```python
from build123d import *

# Parameters (mm, degrees)
SKETCH1_R           = 2.075
SKETCH1_R_2         = 6.003208263
BOSS_EXTRUDE2_DEPTH = 8
FILLET1_R           = 2
CUT_EXTRUDE1_DEPTH  = 10
FILLET2_R           = 2
CUT_EXTRUDE2_DEPTH  = 10
FILLET3_R           = 2


with BuildPart() as part:
    # Sketch1 → Boss-Extrude2 (new body)
    with BuildSketch(Plane(origin=(0, 0, 0), x_dir=(1, 0, 0), z_dir=(0, 1, 0))):
        with BuildLine():
            Line((0, 44.83), (0, 36.83))
            ThreePointArc((0, 36.83), (36.83, 0), (0, -36.83))
            Line((0, -36.83), (0, -46.83))
            Line((0, -46.83), (0, -58.83))
            ThreePointArc((0, -58.83), (14.116701064, -87.229775601), (8, -56.110417137))
            Line((8, -56.110417137), (8, -44.110417137))
            ThreePointArc((8, -44.110417137), (44.649741882, 4.016148637), (0, 44.83))
        make_face()
        with Locations(Location((0.96696537, -64.081170969, 0), (0, 0, 270))):
            Circle(SKETCH1_R, mode=Mode.SUBTRACT)
        with Locations(Location((16.96696537, -64.081170969, 0), (0, 0, 270))):
            Circle(SKETCH1_R, mode=Mode.SUBTRACT)
        with Locations(Location((16.96696537, -80.081170969, 0), (0, 0, 270))):
            Circle(SKETCH1_R, mode=Mode.SUBTRACT)
        with Locations(Location((0.96696537, -80.081170969, 0), (0, 0, 270))):
            Circle(SKETCH1_R, mode=Mode.SUBTRACT)
        with Locations(Location((8.96696537, -72.081170969, 0), (0, 0, 270))):
            Circle(SKETCH1_R_2, mode=Mode.SUBTRACT)
    extrude(amount=BOSS_EXTRUDE2_DEPTH)

    # Fillet1
    fillet1_edges = [part.edges().sort_by_distance(p)[0] for p in [
        (0, 4, 58.83),
        (0, 4, 36.83),
        (0, 4, -36.83),
        (0, 4, -44.83),
        (8, 4, 44.110417137),
        (8, 4, 56.110417137),
    ]]
    fillet(fillet1_edges, radius=FILLET1_R)

    # Sketch2 → Cut-Extrude1 (cut)
    with BuildSketch(Plane(origin=(0, 8, 0), x_dir=(1, 0, 0), z_dir=(0, 1, 0))):
        with BuildLine():
            Line((41.799027506, 16.204018007), (33.073837099, 16.204018007))
            ThreePointArc((33.073837099, 16.204018007), (20.287775905, 30.738494576), (1.896986866, 36.781113915))
            ThreePointArc((1.896986866, 36.781113915), (0.549823068, 37.401147764), (0, 38.778459227))
            Line((0, 38.778459227), (0, 42.783278276))
            Line((0, 42.783278276), (0, 44.783278276))
            Line((0, 44.783278276), (-0.257809332, 46.655742188))
            Line((-0.257809332, 46.655742188), (2.752058537, 46.655742188))
            Line((2.752058537, 46.655742188), (2.752058537, 44.782949944))
            ThreePointArc((2.752058537, 44.782949944), (26.871190964, 36.772449298), (41.799027506, 16.204018007))
        make_face()
    extrude(amount=-CUT_EXTRUDE1_DEPTH, mode=Mode.SUBTRACT)

    # Fillet2
    fillet2_edges = [part.edges().sort_by_distance(p)[0] for p in [
        (41.799027506, 4, -16.204018007),
        (33.073837099, 4, -16.204018007),
    ]]
    fillet(fillet2_edges, radius=FILLET2_R)

    # Sketch3 → Cut-Extrude2 (cut)
    with BuildSketch(Plane(origin=(0, 8, 0), x_dir=(1, 0, 0), z_dir=(0, 1, 0))):
        Polygon((34.701551804, 11.204018007), (33.222316064, 16.570796176), (43.892135876, 17.266509565), (44.733726157, 11.204018007), align=None)
    extrude(amount=-CUT_EXTRUDE2_DEPTH, mode=Mode.SUBTRACT)

    # Fillet3
    fillet3_edges = [part.edges().sort_by_distance(p)[0] for p in [
        (43.40735975, 4, -11.204018007),
        (35.084453544, 4, -11.204018007),
    ]]
    fillet(fillet3_edges, radius=FILLET3_R)


solid = part.part
```
Geometry check sheet. Reference: the model listing, model coordinates, mm. A direction names the side the tool comes from. Coordinates: 2 decimals unless noted, no trailing zeros. Write each loop counter-clockwise with the first axis right and the second up, starting at its lowest first coordinate (ties: lowest second). Pieces come first, ordered by that corner, then holes. Notation, with made-up numbers: M -2.75,29.25 L 42.25,29.25 A31 ccw 42.25,64.25 Z; hole C -11,55.5 d5. An arc over 180 degrees is marked long. Use one line per item in the form item = value. Start each with the question number.
1) Section check A-A on x = 12.5. Enter the section's corners in (y, z).
2) Section check D-D on z = 71.5. Enter the section's corners in (x, y), and give its area (3 significant figures).
3) Go/stop test with flat-tipped pins: pin 1 Ø3 at (x, y) = (30.5, 1) entering from +Z; pin 2 Ø2.5 at (y, z) = (4, 48) entering from -X; pin 3 Ø4 at (y, z) = (5, 25.5) entering from +X. Record where each tip stops, or that it passes through.
4) Section check C-C on x = 20.5. Enter the section's corners in (y, z).
5) Thickness scan on probe 1 along X at (y, z) = (3, 63); probe 2 along Z at (x, y) = (10.5, 6.75); probe 3 along X at (y, z) = (2, 80). Record the ranges inside material, lowest first. Write a range as from..to.
6) Release check for a two-part mould opening along Z. For faces 4 (the cylindrical face through (10.77, 3.944, 77.807)), 5 (the flat face through (13, 8, 42)), 6 (the cylindrical face through (0.56, 4.06, 37.39)) record: pulls with the +Z half, pulls with the -Z half, needs draft (parallel to the pull), parting line crosses it, or undercut.
7) Section check B-B on y = 4.25. Enter the section's corners in (x, z) (3 decimals).
8) Set-up check for faces 1 (the cylindrical face through (18.37, 3.94, 78.55)), 2 (the cylindrical face through (8.454, 4.056, 44.481)), 3 (the flat face through (0, 4, 48)): record each of +Z, -Z, +X, -X, +Y, -Y from which the full face is reachable in a straight line by a thin tool's end or side.
Responses:
q1.outline = M 0,34.64 L 8,34.64 L 8,43.05 L 0,43.05 Z; M 0,56.48 L 8,56.48 L 8,67.23 L 0,67.23 Z; M 0,76.93 L 8,76.93 L 8,87.69 L 0,87.69 Z
q2.outline = M -7.02,0 L 2.99,0 L 2.99,8 L -7.02,8 Z; M 14.94,0 L 24.96,0 L 24.96,8 L 14.94,8 Z
q2.area = 160 mm2
q3.pin_1 = 34.19
q3.pin_2 = 0
q3.pin_3 = 38.18
q4.outline = M 0,30.6 L 8,30.6 L 8,39.87 L 0,39.87 Z; M 0,60.99 L 8,60.99 L 8,83.17 L 0,83.17 Z
q5.probe_1 = -4.21..-0.8, 2.74..15.2, 18.74..22.14
q5.probe_2 = 35.3..43.58, 56.15..66.28, 77.89..88.01
q5.probe_3 = -4.94..-1.11, 3.04..14.89, 19.04..22.87
q6.face_4 = undercut
q6.face_5 = needs draft
q6.face_6 = pulls with the -Z half
q7.outline = M -0.781,59.394 A2 cw 0,57.808 L 0,38.778 A2 ccw 1.897,36.781 A36.83 cw 35.78,-8.73 A2 ccw 37.723,-11.204 L 41.829,-11.204 A2 ccw 43.783,-9.634 A44.83 ccw 9.573,43.796 A2 cw 8,45.75 L 8,54.111 A2 cw 9.885,56.108 A16 ccw long Z; hole C 0.967,64.081 d4.15; hole C 0.967,80.081 d4.15; hole C 8.967,72.081 d12.006; hole C 16.967,64.081 d4.15; hole C 16.967,80.081 d4.15
q8.face_1 = +Y, -Y
q8.face_2 = +X, +Y, -Y
q8.face_3 = -Z, -X, +Y, -Y
